Work out the finished part from the listing and answer in its coordinate system (mm). Face numbers are marked on the shaded views. A direction names the side the tool comes from. Round coordinates to 2 decimals unless told otherwise and drop trailing zeros. Write each loop counter-clockwise with the first axis right and the second up, starting at its lowest first coordinate (ties: lowest second). Pieces come first, ordered by that corner, then holes. Notation, with made-up numbers: (31, 11) - (44, 11) arc R33 ccw to (44, 43) - close; hole circle Ø6 at (-16, 70). An arc over 180 degrees is marked (long way). Answer as a JSON object with one key per item and string values.
```python
from build123d import *

# Parameters (mm, degrees)
SKETCH_1_R          = 8.4
EXTRUDE_1_DEPTH     = 28
SKETCH_2_R          = 7
CUT_EXTRUDE_3_DEPTH = 23
HOLE_WIZARD_M4_1_D  = 3.3
SKETCH_10_R         = 10.4
SKETCH_10_R_2       = 8.4
SKETCH_10_R_3       = 7
EXTRUDE_4_DEPTH     = 1
CHAMFER_1_SIZE      = 0.5


with BuildPart() as part:
    # 草图1 → 凸台-拉伸1 (new body)
    with BuildSketch(Plane.XY):
        Circle(SKETCH_1_R)
    extrude(amount=EXTRUDE_1_DEPTH)

    # 草图2 → 切除-拉伸3 (cut)
    with BuildSketch(Plane.XY.offset(28)):
        Circle(SKETCH_2_R)
    extrude(amount=-CUT_EXTRUDE_3_DEPTH, mode=Mode.SUBTRACT)

    # M4 螺纹孔1 (through all)
    with Locations(Plane(origin=(0, 0, 0), x_dir=(-1, 0, 0), z_dir=(0, 0, -1))):
        with Locations((0, 5), (0, 0), (-4.330127019, -2.5), (4.330127019, -2.5)):
            Hole(HOLE_WIZARD_M4_1_D / 2)

    # 草图10 → 凸台-拉伸4 (add)
    # profile 1 of 2: a face of its own
    with BuildSketch(Plane.XY.offset(28)):
        Circle(SKETCH_10_R)
        Circle(SKETCH_10_R_2, mode=Mode.SUBTRACT)
    # profile 2 of 2: a face of its own
    with BuildSketch(Plane.XY.offset(28)):
        Circle(SKETCH_10_R_2)
        Circle(SKETCH_10_R_3, mode=Mode.SUBTRACT)
    extrude(amount=EXTRUDE_4_DEPTH)

    # 倒角1
    chamfer_1_edges = [part.edges().sort_by_distance(p)[0] for p in [
        (-8.4, 0, 0),
    ]]
    chamfer(chamfer_1_edges, length=CHAMFER_1_SIZE)


solid = part.part
```
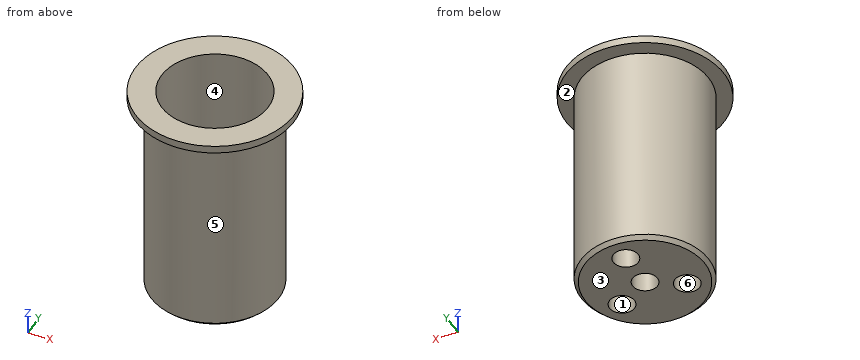
Item 1: Determine the mould class of the marked faces 3, 4, 5 and 6 for opening direction X: pulls with the +X half, pulls with the -X half, needs draft (parallel to the pull), parting line crosses it, or undercut.
Results found:
{"face 3": "needs draft", "face 4": "undercut", "face 5": "parting line crosses it", "face 6": "undercut"}
Item 2: A cutting plane is placed at D-D (z = 8.5). Write down the section's boundary in (x, y), and give its area (3 significant figures).
Results found:
{"outline": "circle Ø16.8 at (0, 0); hole circle Ø14 at (0, 0)", "area": "67.7 mm²"}
Item 3: Consider line 1 along Y through (x, z) = (0, 2.85); line 2 along Z through (x, y) = (-1.5, -5.75); line 3 along Y through (x, z) = (3.25, 4). Determine where each line is inside the solid, lowest interval first.
Results found:
{"line 1": "-8.4 to -1.65, 1.65 to 3.35, 6.65 to 8.4", "line 2": "0 to 5", "line 3": "-7.75 to -3.75, -1.25 to 7.75"}
Item 4: For the marked faces 1 and 2, determine the directions among +Z, -Z, +X, -X, +Y, -Y from which every point of the face is accessible in a straight line to the end or side of a thin tool.
Results found:
{"face 1": "+Z, -Z", "face 2": "-Z"}
Item 5: A cutting plane is placed at C-C (z = 3.75). Write down the section's boundary in (x, y).
Results found:
{"outline": "circle Ø16.8 at (0, 0); hole circle Ø3.3 at (-4.33, -2.5); hole circle Ø3.3 at (0, 0); hole circle Ø3.3 at (0, 5); hole circle Ø3.3 at (4.33, -2.5)"}
Item 6: A cutting plane is placed at B-B (x = 0). Write down the section's boundary in (y, z), and give its area (3 significant figures).
Results found:
{"outline": "(-10.4, 28) - (-8.4, 28) - (-8.4, 0.5) - (-7.9, 0) - (-1.65, 0) - (-1.65, 5) - (-7, 5) - (-7, 29) - (-10.4, 29) - close; (1.65, 0) - (3.35, 0) - (3.35, 5) - (1.65, 5) - close; (6.65, 0) - (7.9, 0) - (8.4, 0.5) - (8.4, 28) - (10.4, 28) - (10.4, 29) - (7, 29) - (7, 5) - (6.65, 5) - close", "area": "122 mm²"}
Item 7: Each of these flat-tipped pins is pushed along its axis until it touches: P1, Ø12, axis at y = -1.5, z = 19.5, coming from the -X side; P2, Ø4, axis at x = 0, y = 0, coming from the +Z side; P3, Ø10, axis at x = -2.5, z = 19.5, coming from the +Y side; P4, Ø2, axis at x = -4.33, y = -2.5, coming from the +Z side. Where does it stop, or does it pass through?
Results found:
{"P1": "x = -8.4", "P2": "z = 5", "P3": "y = 8.4", "P4": "through"}
Item 8: A cutting plane is placed at A-A (y = 0). Write down the section's boundary in (x, z).
Results found:
{"outline": "(-10.4, 28) - (-8.4, 28) - (-8.4, 0.5) - (-7.9, 0) - (-1.65, 0) - (-1.65, 5) - (-7, 5) - (-7, 29) - (-10.4, 29) - close; (1.65, 0) - (7.9, 0) - (8.4, 0.5) - (8.4, 28) - (10.4, 28) - (10.4, 29) - (7, 29) - (7, 5) - (1.65, 5) - close"}
